The model under review builds one solid part; all positions refer to its coordinate system, in mm. A direction names the side the tool comes from. Round coordinates to 2 decimals unless told otherwise and drop trailing zeros. Write each loop counter-clockwise with the first axis right and the second up, starting at its lowest first coordinate (ties: lowest second). Pieces come first, ordered by that corner, then holes. Notation, with made-up numbers: (76, 51) -> (82, 51) arc R29 ccw to (82, 71) -> close; hole circle Ø5 at (45.25, 84.5). An arc over 180 degrees is marked (long way). Use CSV: the item, a comma, the result in double quotes. Start each with the question number.
1) Wall thickness on probe 1 along X at (y, z) = (-24, 604); probe 2 along X at (y, z) = (-13.5, 721); probe 3 along Y at (x, z) = (-23.5, 732): over which ranges is each line inside the solid? List them lowest first. Write a range as [from, to].
2) Take a section at A-A, the plane x = 2. Give the boundary of the cut face in (y, z).
3) Take a section at B-B, the plane y = 1. Give the boundary of the cut face in (x, z), then the cut area to 3 significant figures.
4) For pin 1 Ø14 at (y, z) = (8.5, 747) entering from +X; pin 2 Ø23 at (x, z) = (-5, 765) entering from -Y, all flat-tipped, find the tip position at first contact; note any pin that passes through.
5) Machinability: for faces 1 (the face through (-5, -17.5, 751)), 2 (the face through (0, -28.5, 345)), 3 (the face through (17.5, 6, 751)), which of the approach directions +Z, -Z, +X, -X, +Y, -Y give a long, thin tool a straight path to every point of the face, cutting with its end or side? Answer none if there is none.
from build123d import *

# Parameters (mm, degrees)
F1_DEPTH = 800
F3_DEPTH = 100


with BuildPart() as f1:
    # F0 (on Top) → F1 (new body)
    with BuildSketch(Plane.XY):
        with BuildLine():
            Line((23.5, 28.5), (-23.5, 28.5))
            ThreePointArc((-23.5, 28.5), (-27.035534, 27.035534), (-28.5, 23.5))
            Line((-28.5, 23.5), (-28.5, -23.5))
            ThreePointArc((-28.5, -23.5), (-27.035534, -27.035534), (-23.5, -28.5))
            Line((-23.5, -28.5), (23.5, -28.5))
            ThreePointArc((23.5, -28.5), (27.035534, -27.035534), (28.5, -23.5))
            Line((28.5, -23.5), (28.5, 23.5))
            ThreePointArc((28.5, 23.5), (27.035534, 27.035534), (23.5, 28.5))
        make_face()
    extrude(amount=F1_DEPTH)

    # F2 (on face) → F3 (cut)
    with BuildSketch(Plane.XY.offset(800)):
        Polygon((-35.619496, -17.5), (-35.619496, -32.5), (32.5, -32.5), (32.5, 34.954965), (17.5, 34.954965), (17.5, -17.5), align=None)
    extrude(amount=-F3_DEPTH, mode=Mode.SUBTRACT)


solid = f1.part
Values found:
1,probe 1,"[-28.47, 28.47]"
1,probe 2,"[-28.5, 17.5]"
1,probe 3,"[-17.5, 28.5]"
2,outline,"(-28.5, 0) -> (28.5, 0) -> (28.5, 800) -> (-17.5, 800) -> (-17.5, 700) -> (-28.5, 700) -> close"
3,outline,"(-28.5, 0) -> (28.5, 0) -> (28.5, 700) -> (17.5, 700) -> (17.5, 800) -> (-28.5, 800) -> close"
3,area,"44,500 mm²"
4,pin 1,"x = 17.5"
4,pin 2,"y = -17.5"
5,face 1,"+Z, +X, -X, -Y"
5,face 2,"+Z, -Z, +X, -X, -Y"
5,face 3,"+Z, +X, +Y, -Y"
